CAD build for the part. Positions are in the model's coordinates, mm. Round coordinates to 2 decimals unless told otherwise and drop trailing zeros. Loops run counter-clockwise (first coordinate to the right, second up) from the corner with the lowest first, then second, coordinate; pieces in that order, holes last.
Autodesk Inventor part; units mm, degrees
ref_plane "YZ Plane" through (0, 0, 0) normal (1, 0, 0) x (0, 1, 0)
ref_plane "XZ Plane" through (0, 0, 0) normal (0, 1, 0) x (-1, 0, 0)
ref_plane "XY Plane" through (0, 0, 0) normal (0, 0, 1) x (1, 0, 0)
sketch "Sketch2" plane through (0, 0, 0) normal (0, 0, 1) x (1, 0, 0)
  line L0 (-75, -25) -> (75, -25)
  line L1 (75, -25) -> (75, 25)
  line L2 (75, 25) -> (-75, 25)
  line L3 (-75, 25) -> (-75, -25)
  line L4 (-75, -25) -> (75, 25) construction
  line L5 (75, -25) -> (-75, 25) construction
  point P0 (0, 0)
  dimension "d1" = 150
  dimension "d2" = 50
extrude "Extrusion1" add sketch "Sketch2" along normal mid plane 10
sketch "Sketch3" plane through (0, 0, 5) normal (0, 0, 1) x (1, 0, 0)
  line L0 (-75, 25) -> (-75, -25)
  line L1 (75, 25) -> (-75, 25)
  point P0 (0, 0)
  point P1 (-65, 0)
  dimension "d40" = 10
  dimension "d43" = 25
hole "Hole1" at (-65, 0, 5) direction (0, 0, -1) diameter 4.5 depth 14.2 tip angle 118 counterbore diameter 8 counterbore depth 4.4
sketch "Sketch4" plane through (0, 0, 5) normal (0, 0, 1) x (1, 0, 0)
  line L0 (-75, 25) -> (-75, -25)
  line L1 (75, 25) -> (-75, 25)
  point P0 (0, 0)
  point P1 (-45, 5)
  dimension "d41" = 30
  dimension "d42" = 20
hole "Hole2" at (-45, 5, 5) direction (0, 0, -1) diameter 5.5 depth 14.2 tip angle 118 counterbore diameter 10 counterbore depth 5.4
sketch "Sketch5" plane through (0, 0, 5) normal (0, 0, 1) x (1, 0, 0)
  line L0 (-75, 25) -> (-75, -25)
  line L1 (75, 25) -> (-75, 25)
  point P0 (0, 0)
  point P1 (-25, 5)
  dimension "d44" = 50
  dimension "d45" = 20
hole "Hole3" at (-25, 5, 5) direction (0, 0, -1) diameter 11 depth 14.2 tip angle 118 counterbore diameter 18 counterbore depth 10.8
properties part number "홀간 거리 확인 파트-8" material "SS400"
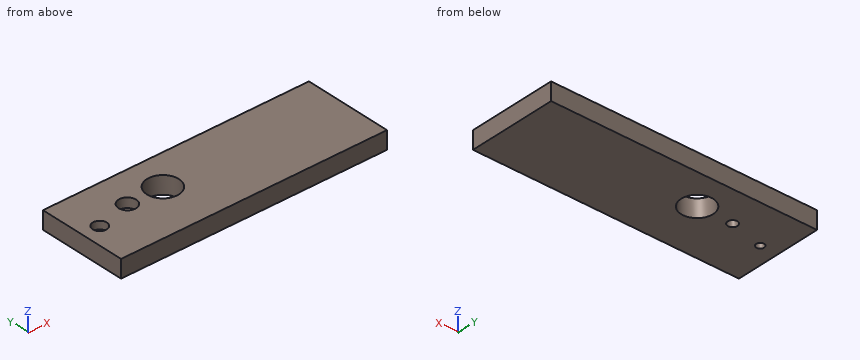
Item 1: Cut at D-D (x = -19). List the corners of the cut face in (y, z).
Verdict:
outline: (-25, -5) - (-1.71, -5) - (-1.71, 5) - (-25, 5) - close; (11.71, -5) - (25, -5) - (25, 5) - (11.71, 5) - close
Item 2: Flat gauge pins, fed straight in: P1, Ø11, axis at x = -46, y = 3.5, coming from the +Z side; P2, Ø5, axis at x = -65, y = 0, coming from the +Z side; P3, Ø16, axis at x = -25, y = 5, coming from the -Z side. Where does each tip first touch, or does it go through?
Verdict:
P1: stops at z = 5
P2: stops at z = 0.6
P3: passes through
Item 3: Wall check: L1, parallel to X at y = 5, z = 3.7; L2, parallel to Y at x = -45, z = -3.3; L3, parallel to Y at x = -25, z = 2.75. Give the ranges that are in metal, low to high.
Verdict:
L1: x = -75 to -50, -40 to -34, -16 to 75
L2: y = -25 to 2.25, 7.75 to 25
L3: y = -25 to -4, 14 to 25
Item 4: Cut at B-B (z = -3). List the corners of the cut face in (x, y).
Verdict:
outline: (-75, -25) - (75, -25) - (75, 25) - (-75, 25) - close; hole circle Ø4.5 at (-65, 0); hole circle Ø5.5 at (-45, 5); hole circle Ø18 at (-25, 5)
Item 5: Cut at A-A (x = -45). List the corners of the cut face in (y, z).
Verdict:
outline: (-25, -5) - (2.25, -5) - (2.25, -0.4) - (0, -0.4) - (0, 5) - (-25, 5) - close; (7.75, -5) - (25, -5) - (25, 5) - (10, 5) - (10, -0.4) - (7.75, -0.4) - close
Item 6: Cut at C-C (y = 12). List the corners of the cut face in (x, z), plus the area to 3 significant figures.
Verdict:
outline: (-75, -5) - (-30.66, -5) - (-30.66, 5) - (-75, 5) - close; (-19.34, -5) - (75, -5) - (75, 5) - (-19.34, 5) - close
area: 1,390 mm2
